CAD build for the part. Positions are in the model's coordinates, mm. A direction names the side the tool comes from. Coordinates: 2 decimals unless noted, no trailing zeros. Order: outer loops, then holes, each group sorted by start corner. A loop starts at its lowest first (then second) coordinate and runs counter-clockwise, first axis right, second up.
from build123d import *

# Parameters (mm, degrees)
SKIZZE2_W                       = 144.44
SKIZZE2_H                       = 77
AUFSATZ_LINEAR_AUSTRAGEN1_DEPTH = 4
SKIZZE4_W                       = 77
SKIZZE4_H                       = 24.6
AUFSATZ_LINEAR_AUSTRAGEN2_DEPTH = 10.6
VERRUNDUNG2_R                   = 6
SKIZZE5_W                       = 47
SKIZZE5_H                       = 53.5
AUFSATZ_LINEAR_AUSTRAGEN3_DEPTH = 14.6
VERRUNDUNG4_R                   = 6
SKIZZE7_R                       = 6.75
AUFSATZ_LINEAR_AUSTRAGEN5_DEPTH = 11.6
WANDUNG2_T                      = -1
SKIZZE8_R                       = 2.5
SCHNITT_LINEAR_AUSTRAGEN1_DEPTH = 84.314694982


with BuildPart() as part:
    # Skizze2 → Aufsatz-Linear austragen1 (new body)
    with BuildSketch(Plane(origin=(0, 0, 0), x_dir=(0, 1, 0), z_dir=(0, 0, 1))):
        Rectangle(SKIZZE2_W, SKIZZE2_H)
    extrude(amount=AUFSATZ_LINEAR_AUSTRAGEN1_DEPTH)

    # Skizze4 → Aufsatz-Linear austragen2 (add)
    with BuildSketch(Plane.XY.offset(4)):
        with Locations((0, -59.92)):
            Rectangle(SKIZZE4_W, SKIZZE4_H)
    extrude(amount=AUFSATZ_LINEAR_AUSTRAGEN2_DEPTH)

    # Verrundung2
    verrundung2_edges = [part.edges().sort_by_distance(p)[0] for p in [
        (38.5, 72.22, 2),
        (38.5, -72.22, 7.3),
        (-38.5, -72.22, 7.3),
        (-38.5, 72.22, 2),
    ]]
    fillet(verrundung2_edges, radius=VERRUNDUNG2_R)

    # Skizze5 → Aufsatz-Linear austragen3 (add)
    with BuildSketch(Plane.XY.offset(4)):
        with Locations((15, 0.03)):
            Rectangle(SKIZZE5_W, SKIZZE5_H)
    extrude(amount=AUFSATZ_LINEAR_AUSTRAGEN3_DEPTH)

    # Verrundung4
    verrundung4_edges = [part.edges().sort_by_distance(p)[0] for p in [
        (38.5, -26.72, 11.3),
        (38.5, 26.78, 11.3),
        (-8.5, 26.78, 11.3),
        (-8.5, -26.72, 11.3),
    ]]
    fillet(verrundung4_edges, radius=VERRUNDUNG4_R)

    # Skizze7 → Aufsatz-Linear austragen5 (add)
    with BuildSketch(Plane.XY.offset(4)):
        with Locations(Location((24.503110224, 58.349132978, 0), (0, 0, 180))):
            Circle(SKIZZE7_R)
    extrude(amount=AUFSATZ_LINEAR_AUSTRAGEN5_DEPTH)

    # Wandung2
    wandung2_openings = [part.faces().sort_by_distance(p)[0] for p in [
        (0, 0, 0),
    ]]
    offset(amount=WANDUNG2_T, openings=wandung2_openings, kind=Kind.INTERSECTION)

    # Skizze8 → Schnitt-Linear austragen1 (cut, through all)
    with BuildSketch(Plane.XY.offset(15.6)):
        with Locations((24.503110224, 58.349132978)):
            Circle(SKIZZE8_R)
    extrude(amount=-SCHNITT_LINEAR_AUSTRAGEN1_DEPTH, mode=Mode.SUBTRACT)


solid = part.part
1) Drill centre lines: probe 1 along Y at (x, z) = (9, 6.25); probe 2 along Y at (x, z) = (28.5, 15); probe 3 along Y at (x, z) = (0.5, 2.75). Where is each one in solid material? Low to high.
2) Pin check, flat tips, straight feed: P1, Ø3, axis at x = -25, y = -48, coming from the -Z side; P2, Ø15, axis at x = 27, y = 61.5, coming from the +Z side; P3, Ø8, axis at y = -40, z = 6.5, coming from the +X side; P4, Ø1, axis at x = -22.5, y = -49.5, coming from the +Z side. Stop position of each tip, or through.
3) Slice it at B-B (y = -61). List the corners of the cut face in (x, z), plus the area to 3 significant figures.
4) Which spindle directions (+Z, -Z, +X, -X, +Y, -Y) get a long thin tool onto all of the face, cutting with end or side? Do faces 4 (the flat face through (0, -72.22, 7)), 5 (the cylindrical face through (22.006, 58.459, 15.107)), 6 (the flat face through (15, 0, 17.6)), 7 (the cylindrical face through (29.48, 53.79, 9.72)), 8 (the cylindrical face through (36.789, -24.916, 11.402)). Say none if no direction does.
5) Slice it at A-A (z = 7.25). Give the number of separate pieces and of enclosed holes in the cut face, plus the area to 3 significant figures.
6) Slice it at D-D (x = 8). List the corners of the cut face in (y, z), plus the area to 3 significant figures.
7) Two-plate mould, pull along Y, no slides. Class faces 1 (the cylindrical face through (36.789, 24.976, 11.402)), 2 (the flat face through (38.5, -1, 7)), 3 (the flat face through (15, -26.72, 11)): released by +Y, released by -Y, zero draft, split by the parting line, or undercut.
Worked out:
1. probe 1: y = -72.22 to -71.22, -48.62 to -47.62, -26.72 to -25.72, 25.78 to 26.78
1. probe 2: y = -26.72 to -25.72, 25.78 to 26.78, 52.91 to 63.79
1. probe 3: y = -72.22 to -71.22, 71.22 to 72.22
2. P1: stops at z = 3
2. P2: stops at z = 15.6
2. P3: stops at x = 38.5
2. P4: stops at z = 14.6
3. outline: (-38.5, 0) - (-37.5, 0) - (-37.5, 13.6) - (37.5, 13.6) - (37.5, 0) - (38.5, 0) - (38.5, 14.6) - (-38.5, 14.6) - close
3. area: 104 mm2
4. face 4: +Z, -Z, +X, -X, -Y
4. face 5: +Z, -Z
4. face 6: -Z
4. face 7: +Z
4. face 8: +Z, +X
5. separate pieces: 3
5. enclosed holes: 3
5. area: 421 mm2
6. outline: (-72.22, 0) - (-71.22, 0) - (-71.22, 13.6) - (-48.62, 13.6) - (-48.62, 3) - (-25.72, 3) - (-25.72, 17.6) - (25.78, 17.6) - (25.78, 3) - (71.22, 3) - (71.22, 0) - (72.22, 0) - (72.22, 4) - (26.78, 4) - (26.78, 18.6) - (-26.72, 18.6) - (-26.72, 4) - (-47.62, 4) - (-47.62, 14.6) - (-72.22, 14.6) - close
6. area: 201 mm2
7. face 1: released by +Y
7. face 2: zero draft
7. face 3: undercut
